Design review of the part built by this model. Coordinates are the model's own, in mm. Face numbers are marked on the shaded views. A direction names the side the tool comes from. Coordinates: 2 decimals unless noted, no trailing zeros. Loops run counter-clockwise (first coordinate to the right, second up) from the corner with the lowest first, then second, coordinate; pieces in that order, holes last. Notation, with made-up numbers: (81, -38.5) -> (118, -38.5) arc R21 ccw to (118, -21.5) -> close; hole circle Ø7 at (-9, 19). An arc over 180 degrees is marked (long way). Use CSV: the item, a comma, the result in double quotes.
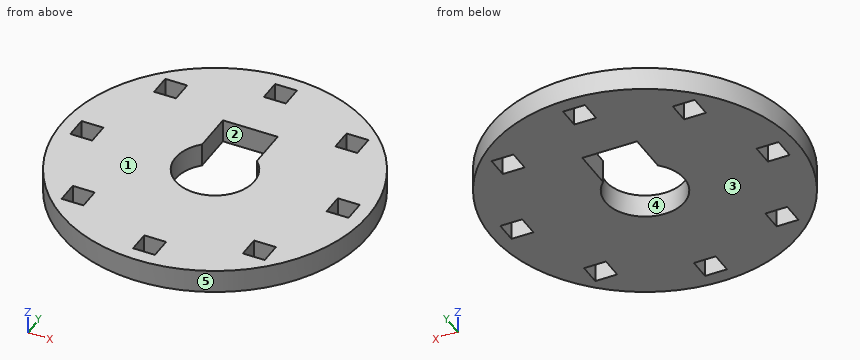
```python
from build123d import *

# Parameters (mm, degrees)
SKETCH1_R           = 20.955
SKETCH1_W           = 2.9972
SKETCH1_H           = 2.9972
BOSS_EXTRUDE1_DEPTH = 3.175
CUT_EXTRUDE1_DEPTH  = 3.175


# Read off the part's stored shape, not the designer's step: Cut-Extrude1
with BuildPart() as part:
    # Sketch1 → Boss-Extrude1 (new body)
    with BuildSketch(Plane.XY):
        Circle(SKETCH1_R)
        with Locations((0, 17.526)):
            Rectangle(SKETCH1_W, SKETCH1_H, mode=Mode.SUBTRACT)
        with Locations((0, -17.526)):
            Rectangle(SKETCH1_W, SKETCH1_H, mode=Mode.SUBTRACT)
        with Locations((17.526, 0)):
            Rectangle(SKETCH1_W, SKETCH1_H, mode=Mode.SUBTRACT)
        with Locations((-17.526, 0)):
            Rectangle(SKETCH1_W, SKETCH1_H, mode=Mode.SUBTRACT)
        with Locations((12.392753447, 12.392753447)):
            Rectangle(SKETCH1_W, SKETCH1_H, mode=Mode.SUBTRACT)
        with Locations((-12.392753447, 12.392753447)):
            Rectangle(SKETCH1_W, SKETCH1_H, mode=Mode.SUBTRACT)
        with Locations((-12.392753447, -12.392753447)):
            Rectangle(SKETCH1_W, SKETCH1_H, mode=Mode.SUBTRACT)
        with Locations((12.392753447, -12.392753447)):
            Rectangle(SKETCH1_W, SKETCH1_H, mode=Mode.SUBTRACT)
    extrude(amount=BOSS_EXTRUDE1_DEPTH)

    # Cut-Extrude1 outline → Cut-Extrude1 (cut)
    with BuildSketch(Plane.XY):
        with BuildLine():
            Line((-3.7465, 9.4615), (-3.7465, 3.885452869))
            ThreePointArc((-3.7465, 3.885452869), (0, -5.3975), (3.7465, 3.885452869))
            Line((3.7465, 3.885452869), (3.7465, 9.4615))
            Line((3.7465, 9.4615), (-3.7465, 9.4615))
        make_face()
    extrude(amount=CUT_EXTRUDE1_DEPTH, mode=Mode.SUBTRACT)


solid = part.part
```
Item 1: Draft analysis for pull direction Y (two halves, no side actions). For the marked faces 3, 4 and 5, state which applies: pulls with the +Y half, pulls with the -Y half, needs draft (parallel to the pull), parting line crosses it, or undercut.
Checked values:
face 3,"needs draft"
face 4,"undercut"
face 5,"parting line crosses it"
Item 2: Machinability: for the marked faces 1 and 2, which of the approach directions +Z, -Z, +X, -X, +Y, -Y give a long, thin tool a straight path to every point of the face, cutting with its end or side? Answer none if there is none.
Checked values:
face 1,"+Z, +X, -X, +Y, -Y"
face 2,"+Z, -Z"
Item 3: Add section C-C (y = -13). Give the boundary of the cut face in (x, z) (3 decimals).
Checked values:
outline,"(-16.435, 0) -> (-13.891, 0) -> (-13.891, 3.175) -> (-16.435, 3.175) -> close; (-10.894, 0) -> (10.894, 0) -> (10.894, 3.175) -> (-10.894, 3.175) -> close; (13.891, 0) -> (16.435, 0) -> (16.435, 3.175) -> (13.891, 3.175) -> close"
Item 4: Add section B-B (x = 0). Give the boundary of the cut face in (y, z) (1 decimal), then the cut area to 3 significant figures.
Checked values:
outline,"(-21, 0) -> (-19, 0) -> (-19, 3.2) -> (-21, 3.2) -> close; (-16, 0) -> (-5.4, 0) -> (-5.4, 3.2) -> (-16, 3.2) -> close; (9.5, 0) -> (16, 0) -> (16, 3.2) -> (9.5, 3.2) -> close; (19, 0) -> (21, 0) -> (21, 3.2) -> (19, 3.2) -> close"
area,"66.9 mm^2"
Item 5: To check wall thickness, follow line 1 along Y through (x, z) = (0, 2.1) (1 decimal); line 2 along Y through (x, z) = (2, 1.55); line 3 along X through (y, z) = (8, 2.6). State the ranges of each line that lie inside material, in increasing order.
Checked values:
line 1,"-21 to -19, -16 to -5.4, 9.5 to 16, 19 to 21"
line 2,"-20.86 to -5.01, 9.46 to 20.86"
line 3,"-19.37 to -3.75, 3.75 to 19.37"
Item 6: Add section A-A (y = 0). Give the boundary of the cut face in (x, z) (1 decimal).
Checked values:
outline,"(-21, 0) -> (-19, 0) -> (-19, 3.2) -> (-21, 3.2) -> close; (-16, 0) -> (-5.4, 0) -> (-5.4, 3.2) -> (-16, 3.2) -> close; (5.4, 0) -> (16, 0) -> (16, 3.2) -> (5.4, 3.2) -> close; (19, 0) -> (21, 0) -> (21, 3.2) -> (19, 3.2) -> close"
Item 7: Add section D-D (x = -17.5). Give the boundary of the cut face in (y, z) (3 decimals), then the cut area to 3 significant figures.
Checked values:
outline,"(-11.527, 0) -> (-1.499, 0) -> (-1.499, 3.175) -> (-11.527, 3.175) -> close; (1.499, 0) -> (11.527, 0) -> (11.527, 3.175) -> (1.499, 3.175) -> close"
area,"63.7 mm^2"
Item 8: Clearance check with flat-ended pins moving along their axes: pin 1 (0.9 mm diameter, centred on x = 0, z = 1.5, fed in from +Y) (3 decimals); pin 2 (0.9 mm diameter, centred on y = -12.5, z = 1.5, fed in from -X); pin 3 (1 mm diameter, centred on y = -5, z = 0.5, fed in from +X). State where each tip first meets the part, or that it passes through.
Checked values:
pin 1,"y = 20.955"
pin 2,"x = -17.14"
pin 3,"x = 20.47"
